Input: part model. Units: mm. Frame: model coordinates. Face numbers are marked on the shaded views. Round coordinates to 2 decimals unless told otherwise and drop trailing zeros. Loops run counter-clockwise (first coordinate to the right, second up) from the corner with the lowest first, then second, coordinate; pieces in that order, holes last.
(1) Cut plane A-A, the plane z = 11. Give the number of separate pieces and of enclosed holes in the cut face, and give its area (3 significant figures).
(2) Draft query along Z for the marked faces 1 and 2. Return one class per face: released by +Z, released by -Z, zero draft, split by the parting line, or undercut.
(3) First-contact query: pin 1 Ø25 at (x, z) = (-4, -8.5) entering from -Y; pin 2 Ø12 at (x, y) = (-3.5, 38.5) entering from -Z; pin 3 Ø11 at (x, y) = (0, 38) entering from +Z; pin 4 Ø1 at (x, y) = (-8.5, 21.5) entering from -Z. Flat tips, straight axial feed; report the tip coordinate or a pass-through.
(4) Line query: line 1 (X direction, y = 59.8, z = 0); line 2 (Z direction, x = 0, y = 52); line 3 (X direction, y = 49.5, z = 0). Output: solid intervals per line, ascending.
(5) Cut plane B-B, the plane y = 38. Output: boundary loops of the cut face in (x, z).
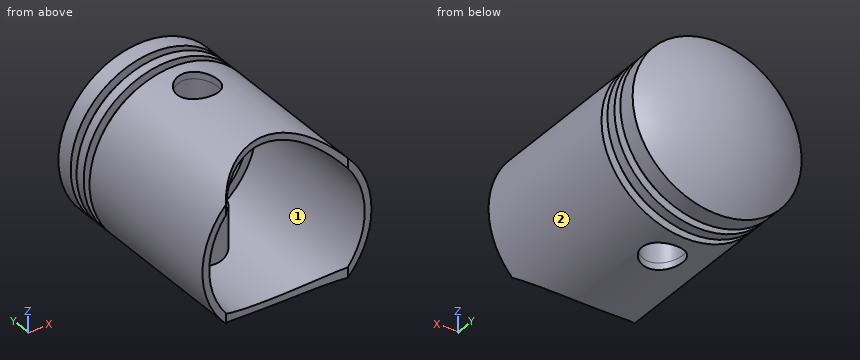
from build123d import *

# Parameters (mm, degrees)
SKETCH2_W                = 2.5
SKETCH2_H                = 2.5
LPATTERN2_COUNT          = 2
LPATTERN2_PITCH          = 5.5
CUT_EXTRUDE1_DEPTH       = 79.421935707
CUT_EXTRUDE1_DEPTH_BACK  = 79.421935707
CUT_EXTRUDE2_DEPTH       = 79.421935771
CUT_EXTRUDE2_DEPTH_BACK  = 79.421935771
SKETCH4_R                = 6
BOSS_EXTRUDE4_REACH      = 90.422
BOSS_EXTRUDE4_END_RADIUS = 23
BOSS_EXTRUDE4_START      = 10
SKETCH5_R                = 7.5
SKETCH5_R_2              = 6


# Read off the part's stored shape, not the designer's step: Shell1
with BuildPart() as part:
    # Sketch1 → Revolve1 (revolve)
    with BuildSketch(Plane.XY):
        with BuildLine():
            Line((0, 0), (0, 70))
            ThreePointArc((0, 70), (13.247648854, 67.742546282), (25, 61.224989992))
            Line((25, 61.224989992), (25, 0))
            Line((25, 0), (0, 0))
        make_face()
    revolve(axis=Axis((0, 0, 0), (0, 1, 0)))

    # Sketch2 → Cut-Revolve2 (revolve, cut)
    with BuildSketch(Plane.XY, mode=Mode.PRIVATE) as cut_revolve2_sk:
        with Locations((23.75, 49.25)):
            Rectangle(SKETCH2_W, SKETCH2_H)
    cut_revolve2 = revolve(cut_revolve2_sk.sketch.rotate(Axis((0, 79.863110142, 0), (0, 1, 0)), 90), axis=Axis((0, 79.863110142, 0), (0, 1, 0)), mode=Mode.SUBTRACT)

    # LPattern2: Cut-Revolve2 ×2
    with Locations(*[(0, i * LPATTERN2_PITCH, 0) for i in range(1, LPATTERN2_COUNT)]):
        add(cut_revolve2, mode=Mode.SUBTRACT)

    # Shell1 outline → Shell1 (revolve, cut)
    with BuildSketch(Plane.XY):
        with BuildLine():
            Line((0, 0), (23, 0))
            Line((23, 0), (23, 46))
            Line((23, 46), (20.5, 46))
            Line((20.5, 46), (20.5, 58))
            Line((20.5, 58), (23, 58))
            Line((23, 58), (23.00000001, 60.248966917))
            ThreePointArc((23.00000001, 60.248966917), (12.135469854, 66.010142619), (0, 68))
            Line((0, 68), (0, 0))
        make_face()
    revolve(axis=Axis((0, 0, 0), (0, 1, 0)), mode=Mode.SUBTRACT)

    # Sketch3 → Cut-Extrude1 (cut, two sides: drawn at the far end of the back side and taken through both)
    with BuildSketch(Plane.XY.offset(-CUT_EXTRUDE1_DEPTH_BACK)):
        with BuildLine():
            Line((-110.085446515, -147.994467613), (-18, 0))
            ThreePointArc((-18, 0), (0, 10), (18, 0))
            Line((18, 0), (110.085446515, -147.994467613))
            Line((110.085446515, -147.994467613), (110.085446515, -496.603657989))
            Line((110.085446515, -496.603657989), (-110.085446515, -496.603657989))
            Line((-110.085446515, -496.603657989), (-110.085446515, -147.994467613))
        make_face()
    extrude(amount=CUT_EXTRUDE1_DEPTH + CUT_EXTRUDE1_DEPTH_BACK, mode=Mode.SUBTRACT)

    # Sketch4 → Cut-Extrude2 (cut, two sides: drawn at the far end of the back side and taken through both)
    with BuildSketch(Plane.XY.offset(-CUT_EXTRUDE2_DEPTH_BACK)):
        with Locations((0, 38)):
            Circle(SKETCH4_R)
    extrude(amount=CUT_EXTRUDE2_DEPTH + CUT_EXTRUDE2_DEPTH_BACK, mode=Mode.SUBTRACT)

    # Boss-Extrude4: up to this cylinder (the profile starts inside it)
    boss_extrude4_end = Plane(origin=(0, 38, 0), z_dir=(0, -1, 0)) * Cylinder(BOSS_EXTRUDE4_END_RADIUS, 227.844, mode=Mode.PRIVATE)
    # Sketch5 → Boss-Extrude4 (add, up to the surface)
    with BuildSketch(Plane.XY.offset(BOSS_EXTRUDE4_START), mode=Mode.PRIVATE) as boss_extrude4_sk1:
        with Locations(Location((0, 38, 0), (0, 0, 180))):
            Circle(SKETCH5_R)
        with Locations((0, 38)):
            Circle(SKETCH5_R_2, mode=Mode.SUBTRACT)
    boss_extrude4_tool1 = extrude(boss_extrude4_sk1.sketch, amount=BOSS_EXTRUDE4_REACH, mode=Mode.PRIVATE) & boss_extrude4_end
    boss_extrude4 = boss_extrude4_tool1.solids().sort_by_distance((7.287868, 38, 10))[0]
    add(boss_extrude4)

    # Mirror1: Boss-Extrude4 across plane
    add(boss_extrude4.mirror(Plane.XY))


solid = part.part
Reported:
1. separate pieces: 2
1. enclosed holes: 1
1. area: 473 mm2
2. face 1: undercut
2. face 2: split by the parting line
3. pin 1: stops at y = 30.5
3. pin 2: stops at z = -24.98
3. pin 3: passes through
3. pin 4: stops at z = -23.69
4. line 1: x = -25 to -23, 23 to 25
4. line 2: z = -25 to -20.5, 20.5 to 25
4. line 3: x = -22.5 to -20.5, 20.5 to 22.5
5. outline: (-7.5, -21.74) arc R23 cw to (-7.5, 21.74) - (-7.5, 10) - (-6, 10) - (-6, 24.27) arc R25 ccw to (-6, -24.27) - (-6, -10) - (-7.5, -10) - close; (6, -24.27) arc R25 ccw to (6, 24.27) - (6, 10) - (7.5, 10) - (7.5, 21.74) arc R23 cw to (7.5, -21.74) - (7.5, -10) - (6, -10) - close
